Autodesk Inventor part; units mm, degrees
ref_plane "YZ Plane" through (0, 0, 0) normal (1, 0, 0) x (0, 1, 0)
ref_plane "XZ Plane" through (0, 0, 0) normal (0, 1, 0) x (-1, 0, 0)
ref_plane "XY Plane" through (0, 0, 0) normal (0, 0, 1) x (1, 0, 0)
sketch "Sketch1" plane through (0, 0, 0) normal (0, 0, 1) x (1, 0, 0)
  line L0 (55.125, -6.9417) -> (55.125, -0.9417)
  line L1 (55.125, -6.9417) -> (66.5, -6.9417)
  line L2 (66.5, 3.0583) -> (66.5, -6.9417)
  line L3 (66.5, 3.0583) -> (-66.5, 3.0583)
  line L4 (-66.5, -6.9417) -> (-66.5, 3.0583)
  line L5 (-66.5, -6.9417) -> (-55.125, -6.9417)
  line L6 (-55.125, -0.9417) -> (-55.125, -6.9417)
  line L7 (55.125, -0.9417) -> (-55.125, -0.9417)
  line L8 (-55.125, -6.9417) -> (-55.125, -35.9417)
  line L9 (-55.125, -6.9417) -> (-66.5, -6.9417)
  line L10 (-66.5, -40.9417) -> (-66.5, -6.9417)
  line L11 (-37.5645, -40.9417) -> (-66.5, -40.9417)
  line L12 (-37.5645, -38.4017) -> (-37.5645, -40.9417)
  line L13 (-37.5645, -38.4017) -> (-28.75, -38.4017)
  line L14 (55.125, -35.9417) -> (55.125, -6.9417)
  line L15 (28.75, -38.4017) -> (37.5645, -38.4017)
  line L16 (37.5645, -40.9417) -> (37.5645, -38.4017)
  line L17 (66.5, -40.9417) -> (37.5645, -40.9417)
  line L18 (66.5, -6.9417) -> (66.5, -40.9417)
  line L19 (55.125, -6.9417) -> (66.5, -6.9417)
  line L20 (-66.5, 3.0583) -> (-55.125, 3.0583)
  line L21 (-55.125, 3.0583) -> (-55.125, -16.9417)
  line L22 (-55.125, -16.9417) -> (-66.5, -16.9417)
  line L23 (-66.5, -16.9417) -> (-66.5, 3.0583)
  line L24 (-66.5, -6.9417) -> (-66.5, -11.9417)
  circle A0 centre (-60.8125, -1.9417) radius 1.5
  circle A1 centre (-60.8125, -11.9417) radius 1.5
  circle A2 centre (-60.8125, -11.9417) radius 1.375
  circle A3 centre (60.8125, -11.9417) radius 1.375
  circle A4 centre (-60.8125, -1.9417) radius 1.375
  circle A5 centre (60.8125, -1.9417) radius 1.375
  line L25 (-53.125, -37.9417) -> (-28.75, -37.9417)
  arc A6 (-55.125, -35.9417) -> (-53.125, -37.9417) centre (-53.125, -35.9417) ccw
  line L26 (-28.75, -37.9417) -> (-28.75, -38.4017)
  line L27 (28.75, -37.9417) -> (53.125, -37.9417)
  line L28 (28.75, -38.4017) -> (28.75, -37.9417)
  arc A7 (53.125, -37.9417) -> (55.125, -35.9417) centre (53.125, -35.9417) ccw
  point P0 (0, 0)
  point P1 (-60.8125, 3.0583)
  point P2 (-66.5, -1.9417)
  dimension "d0" = 20
  dimension "d1" = 5
  dimension "d2" = 3
  dimension "d4" = 3
extrude "Extrusion1" add sketch "Sketch1" along normal blind 0.5 contours L6 L5 L4 L3 L21 | L8 L22 L10 L5
fillet "Fillet1" radius 2 4 edges at (-66.5, 3.0583, 0.25) (-55.125, 3.0583, 0.25) (-55.125, -16.9417, 0.25) (-66.5, -16.9417, 0.25)
properties part number "FlexHinge"
Input: part model. Units: mm. Frame: model coordinates. Coordinates: 2 decimals unless noted, no trailing zeros. Loops run counter-clockwise (first coordinate to the right, second up) from the corner with the lowest first, then second, coordinate; pieces in that order, holes last. Notation, with made-up numbers: (73.5, 71) -> (125.5, 71) arc R17 cw to (125.5, 92) -> close; hole circle Ø2 at (73.5, 75.25). An arc over 180 degrees is marked (long way). Write item = value, one per line. Start each with the question number.
Item 1: Cut plane A-A, the plane y = -2.5. Return loops of the section in (x, z) (3 decimals).
Item 2: Mould query, pull axis X, two halves, no side actions, for faces 1 (the face through (-65.899, 2.488, 0.254)), 2 (the face through (-59.427, -11.367, 0.246)), 3 (the face through (-61, -7, 0.5)), 4 (the face through (-59.38, -2.39, 0.25)). Classes: pulls with the +X half, pulls with the -X half, needs draft (parallel to the pull), parting line crosses it, or undercut.
Item 3: First-contact query: P1, Ø1.8, axis at x = -60.81, y = -11.94, coming from the -Z side. Flat tip, straight axial feed; report the tip coordinate or a pass-through.
Item 4: Cut plane B-B, the plane z = 0.4. Return loops of the section in (x, y) (1 decimal).
Item 5: Cut plane C-C, the plane x = -60.5. Return loops of the section in (y, z), plus the area to 3 significant figures.
Item 6: Material intervals for line 1 (Y direction, x = -61.25, z = 0.15); line 2 (X direction, y = -3.25, z = 0.1) (3 decimals); line 3 (X direction, y = -11.5, z = 0.4) (3 decimals), sorted ascending.
Item 7: Cut plane D-D, the plane y = -11. Return loops of the section in (x, z) (3 decimals).
Ans:
q1.outline = (-66.5, 0) -> (-62.205, 0) -> (-62.205, 0.5) -> (-66.5, 0.5) -> close; (-59.42, 0) -> (-55.125, 0) -> (-55.125, 0.5) -> (-59.42, 0.5) -> close
q2.face_1 = pulls with the -X half
q2.face_2 = undercut
q2.face_3 = needs draft
q2.face_4 = undercut
q3.P1 = through
q4.outline = (-66.5, -14.9) arc R2 ccw to (-64.5, -16.9) -> (-57.1, -16.9) arc R2 ccw to (-55.1, -14.9) -> (-55.1, 1.1) arc R2 ccw to (-57.1, 3.1) -> (-64.5, 3.1) arc R2 ccw to (-66.5, 1.1) -> close; hole circle Ø3 at (-60.8, -11.9); hole circle Ø3 at (-60.8, -1.9)
q5.outline = (-16.94, 0) -> (-13.41, 0) -> (-13.41, 0.5) -> (-16.94, 0.5) -> close; (-10.47, 0) -> (-3.41, 0) -> (-3.41, 0.5) -> (-10.47, 0.5) -> close; (-0.47, 0) -> (3.06, 0) -> (3.06, 0.5) -> (-0.47, 0.5) -> close
q5.area = 7.07 mm²
q6.line_1 = -16.94 to -13.38, -10.51 to -3.38, -0.51 to 3.06
q6.line_2 = -66.5 to -61.546, -60.079 to -55.125
q6.line_3 = -66.5 to -62.246, -59.379 to -55.125
q7.outline = (-66.5, 0) -> (-61.98, 0) -> (-61.98, 0.5) -> (-66.5, 0.5) -> close; (-59.645, 0) -> (-55.125, 0) -> (-55.125, 0.5) -> (-59.645, 0.5) -> close
